Autodesk Inventor part; units mm, degrees
ref_plane "Płaszczyzna konstrukcyjna2" through (-60, 15.9, 10) normal (1, 0, 0) x (0, -1, 0)
ref_plane "YZ Plane" through (0, 0, 0) normal (1, 0, 0) x (0, 1, 0)
ref_plane "XZ Plane" through (0, 0, 0) normal (0, 1, 0) x (-1, 0, 0)
sketch "Szkic1" plane through (0, 0, 0) normal (0, 0, 1) x (1, 0, 0)
  circle A0 centre (0, 0) radius 3.5
  circle A1 centre (0, 0) radius 15.9
  circle A2 centre (0, 0) radius 11.5
  line L0 (0, -15.9) -> (-60, -15.9)
  line L1 (0, 15.9) -> (-60, 15.9)
  line L2 (-60, 15.9) -> (-60, -15.9)
  point P0 (0, 7.1)
  point P1 (-7.1, 0)
  point P2 (7.1, 0)
  point P3 (0, -7.1)
  dimension "d0" = 7
  dimension "d1" = 7.1
  dimension "d2" = 7.1
  dimension "d3" = 7.1
  dimension "d4" = 7.1
  dimension "d5" = 31.8
  dimension "d6" = 23
  dimension "d23" = 60
extrude "Wyciągnięcie proste1" add sketch "Szkic1" along normal blind 10 contours A0 | A1 | A1 L0 L2 L1 | A2
extrude "Wyciągnięcie proste2" cut sketch "Szkic1" along normal blind 2 contours A2
extrude "Wyciągnięcie proste3" cut sketch "Szkic1" along normal blind 3 contours A0
hole "Otwór1" at (0, 7.1, 0) at (-7.1, 0, 0) at (7.1, 0, 0) at (0, -7.1, 0) direction (0, 0, 1) diameter 1.567 end through all
sketch "Szkic2" plane through (0, 0, 0) normal (0, 0, -1) x (0, -1, 0)
  arc A0 (-15.9, 0) -> (15.9, 0) centre (0, 0) ccw
  circle A1 centre (0, 0) radius 11.5
  circle A2 centre (0, 0) radius 13.9
  line L0 (15.9, 60) -> (15.9, 0)
  line L1 (-15.9, 60) -> (15.9, 60)
  line L2 (-15.9, 0) -> (-15.9, 60)
  dimension "d20" = 2
extrude "Wyciągnięcie proste4" add sketch "Szkic2" along normal blind 3 contours L2 L1 L0 A0
ref_plane "Płaszczyzna konstrukcyjna2" through (-60, 15.9, 10) normal (1, 0, 0) x (0, -1, 0)
mirror "Odbij1" about plane through (-60, 15.9, 0) normal (-1, 0, 0) of "Wyciągnięcie proste4", "Otwór1", "Wyciągnięcie proste1", "Wyciągnięcie proste2"
sketch "Szkic4" plane through (-120, 0, 0) normal (0, 0, -1) x (-1, 0, 0)
  circle A0 centre (0, 0) radius 3.5
  point P0 (-120, 0)
extrude "Wyciągnięcie proste5" cut sketch "Szkic4" against normal blind 3
sketch "Szkic5" plane through (0, 0, 10) normal (0, 0, 1) x (1, 0, 0)
  circle A0 centre (-127.1, 0) radius 0.7835
  circle A1 centre (-120, -7.1) radius 0.7835
  circle A2 centre (-112.9, 0) radius 0.7835
  circle A3 centre (-120, 7.1) radius 0.7835
  circle A4 centre (7.1, 0) radius 0.7835
  circle A5 centre (0, 7.1) radius 0.7835
  circle A6 centre (-7.1, 0) radius 0.7835
  circle A7 centre (0, -7.1) radius 0.7835
  arc A8 (0, -15.9) -> (0, 15.9) centre (0, 0) ccw
  line L0 (0, 15.9) -> (-120, 15.9)
  arc A9 (-120, 15.9) -> (-120, -15.9) centre (-120, 0) ccw
  line L1 (0, -15.9) -> (-120, -15.9)
  circle A10 centre (0, 7.1) radius 2.5
  circle A11 centre (7.1, 0) radius 2.5
  circle A12 centre (0, -7.1) radius 2.5
  circle A13 centre (-7.1, 0) radius 2.5
  circle A14 centre (-120, 7.1) radius 2.5
  circle A15 centre (-112.9, 0) radius 2.5
  circle A16 centre (-120, -7.1) radius 2.5
  circle A17 centre (-127.1, 0) radius 2.5
  dimension "d27" = 5
  dimension "d28" = 5
  dimension "d29" = 5
  dimension "d30" = 5
  dimension "d31" = 5
  dimension "d32" = 5
  dimension "d33" = 5
  dimension "d34" = 5
extrude "Wyciągnięcie proste6" cut sketch "Szkic5" against normal blind 6 contours A0 | A1 | A2 | A3 | A4 | A5 | A6 | A7 | A10 | A11 | A12 | A13 | A14 | A15 | A16 | A17
equation "\"d18\" = d1"
properties part number "Ramie2_Drukowanie 3D"
For this review, take the finished solid that the model builds, in its own axes (mm). A direction names the side the tool comes from. Coordinates: 2 decimals unless noted, no trailing zeros. Answer as CSV lines item,"result". Start each with the question number.
1) To check wall thickness, follow line 1 along Y through (x, z) = (0, 8.75); line 2 along X through (y, z) = (0, 3.1); line 3 along Y through (x, z) = (-120.5, 2.75). State the ranges of each line that lie inside material, in increasing order. Write a range as [from, to].
2) Add section A-A (z = 6.5). Count the separate pieces of the cut face and the enclosed holes in it, then the cut area to 3 significant figures.
3) Insertion check: P1, Ø1.5, axis at y = -10.5, z = 7.5, coming from the +X side; P2, Ø8, axis at x = 0, y = -7.1, coming from the -Z side; P3, Ø4, axis at y = -6, z = 5.5, coming from the -X side. Each pin has a flat end and moves straight along its axis. Give the tip position at first contact, or say it passes through.
4) Draft analysis for pull direction Y (two halves, no side actions). For faces 1 (the flat face through (-61, -15.9, 4)), 2 (the cylindrical face through (15.896, -0.35, 3.591)), 3 (the cylindrical face through (-0.33, -4.62, 7.04)), state which applies: +Y half, -Y half, draft (parallel to the pull), parting line (faces both ways), or undercut.
5) Machinability: for faces 4 (the flat face through (-61, 0, 10)), 5 (the cylindrical face through (-117.615, -6.349, 7.042)), 6 (the cylindrical face through (3.233, 1.341, 2.493)), which of the approach directions +Z, -Z, +X, -X, +Y, -Y give a long, thin tool a straight path to every point of the face, cutting with its end or side? Answer none if there is none.
Result:
1,line 1,"[-15.9, -9.6], [-4.6, 4.6], [9.6, 15.9]"
1,line 2,"[-135.9, -127.88], [-126.32, -113.68], [-112.12, -7.88], [-6.32, 6.32], [7.88, 15.9]"
1,line 3,"[-15.89, -7.7], [-6.5, -3.46], [3.46, 6.5], [7.7, 15.89]"
2,separate pieces,"1"
2,enclosed holes,"8"
2,area,"4,450 mm^2"
3,P1,"x = 12.56"
3,P2,"z = 2"
3,P3,"x = -135.39"
4,face 1,"-Y half"
4,face 2,"parting line"
4,face 3,"undercut"
5,face 4,"+Z, +X, -X, +Y, -Y"
5,face 5,"+Z"
5,face 6,"-Z"
